```python
from build123d import *

# Parameters (mm, degrees)
F0_W     = 30.243722
F0_H     = 12.7
F1_DEPTH = 254
F2_DEPTH = 25.4


with BuildPart() as f1:
    # F0 (on Top) → F1 (new body)
    with BuildSketch(Plane.XY):
        with BuildLine():
            add(Edge.make_bspline(
                [(-7.819359, 19.657847), (0, 28.573312), (3.134033, 33.92129), (17.580641, 32.357847)],
                knots=[0, 0, 0, 0, 28.398063, 28.398063, 28.398063, 28.398063], degree=3))
            Line((-7.819359, 19.657847), (17.580641, 19.657847))
            Line((17.580641, 19.657847), (17.580641, 32.357847))
        make_face()
        Polygon((17.580641, 19.657847), (-7.819359, 19.657847), (-7.819359, -21.92727), (17.580641, -21.92727), (17.580641, -16.079364), align=None)
        with Locations((32.702502, 26.007847)):
            Rectangle(F0_W, F0_H)
        with BuildLine():
            Line((17.580641, -21.92727), (-7.819359, -21.92727))
            add(Edge.make_bspline(
                [(-7.819359, -21.92727), (-5.692848, -35.277039), (4.585292, -34.272849), (17.580641, -34.62727)],
                knots=[0, 0, 0, 0, 28.398063, 28.398063, 28.398063, 28.398063], degree=3))
            Line((17.580641, -34.62727), (17.580641, -21.92727))
        make_face()
        with Locations((32.702502, -28.27727)):
            Rectangle(F0_W, F0_H)
    extrude(amount=F1_DEPTH)

    # F1_face (on face) → F2 (join)
    with BuildSketch(Plane(origin=(14.443133, -1.495159, 254), x_dir=(1, 0, 0), z_dir=(0, 0, 1))):
        with BuildLine():
            add(Edge.make_bspline(
                [(-22.262492, 21.153006), (-14.443133, 30.068472), (-11.3091, 35.416449), (3.137508, 33.853006)],
                knots=[0, 0, 0, 0, 28.398063, 28.398063, 28.398063, 28.398063], degree=3))
            Line((-22.262492, 21.153006), (-22.262492, -20.432111))
            add(Edge.make_bspline(
                [(-22.262492, -20.432111), (-20.135981, -33.781879), (-9.857842, -32.77769), (3.137508, -33.132111)],
                knots=[0, 0, 0, 0, 28.398063, 28.398063, 28.398063, 28.398063], degree=3))
            Line((3.137508, -33.132111), (33.381229, -33.132111))
            Line((33.381229, -33.132111), (33.381229, -20.432111))
            Line((33.381229, -20.432111), (3.137508, -20.432111))
            Line((3.137508, -20.432111), (3.137508, 21.153006))
            Line((3.137508, 21.153006), (33.381229, 21.153006))
            Line((33.381229, 21.153006), (33.381229, 33.853006))
            Line((33.381229, 33.853006), (3.137508, 33.853006))
        make_face()
    extrude(amount=F2_DEPTH)


solid = f1.part
```
The model under review builds one solid part; all positions refer to its coordinate system, in mm. A direction names the side the tool comes from. Round coordinates to 2 decimals unless told otherwise and drop trailing zeros. Loops run counter-clockwise (first coordinate to the right, second up) from the corner with the lowest first, then second, coordinate; pieces in that order, holes last.
Item 1: For line 1 (Y direction, x = 36, z = 224.5); line 2 (X direction, y = -4.5, z = 250.5); line 3 (Y direction, x = 17.5, z = 152.5), list the stretches that pass through material, from the lowest coordinate up.
Determined:
line 1: y = -34.63 to -21.93, 19.66 to 32.36
line 2: x = -7.82 to 17.58
line 3: y = -34.63 to 32.37
Item 2: Mouldability with a two-part tool opening along Y and no side actions: class faces 3 (the face through (33, 32.358, 138)), 4 (the face through (-7.819, -1, 138)), 5 (the face through (32, -34.627, 138)), 6 (the face through (33, -21.927, 138)) as released by +Y, released by -Y, zero draft, split by the parting line, or undercut.
Determined:
face 3: released by +Y
face 4: zero draft
face 5: released by -Y
face 6: undercut
Item 3: Take a section at A-A (x = 22). Write out the cut boundary in (y, z), then the cut area to 3 significant figures.
Determined:
outline: (-34.63, 0) - (-21.93, 0) - (-21.93, 279.4) - (-34.63, 279.4) - close; (19.66, 0) - (32.36, 0) - (32.36, 279.4) - (19.66, 279.4) - close
area: 7,100 mm2
Item 4: Clearance check with flat-ended pins moving along their axes: pin 1 Ø3 at (x, z) = (29.5, 150) entering from +Y; pin 2 Ø21 at (y, z) = (-9.5, 85.5) entering from +X; pin 3 Ø4 at (x, z) = (-2, 234) entering from -Y. State where each tip first meets the part, or that it passes through.
Determined:
pin 1: stops at y = 32.36
pin 2: stops at x = 17.58
pin 3: stops at y = -32.86
Item 5: For faces 1 (the face through (32, 19.658, 138)), 2 (the face through (47.824, -28, 125)), list the 3-axis set-ups (+Z, -Z, +X, -X, +Y, -Y) from which the entire face can be reached by the end or side of a thin tool; tool diameter is ignored.
Determined:
face 1: +Z, -Z, +X
face 2: +Z, -Z, +X, +Y, -Y
Item 6: Take a section at B-B (y = -13). Write out the cut boundary in (x, z), then the cut area to 3 significant figures.
Determined:
outline: (-7.82, 0) - (17.58, 0) - (17.58, 279.4) - (-7.82, 279.4) - close
area: 7,100 mm2
